Geometry check sheet. Reference: the model listing, model coordinates, mm. A direction names the side the tool comes from. Round coordinates to 2 decimals unless told otherwise and drop trailing zeros. Loops run counter-clockwise (first coordinate to the right, second up) from the corner with the lowest first, then second, coordinate; pieces in that order, holes last. Notation, with made-up numbers: (-5.75, 6) -> (23.25, 6) arc R15 ccw to (23.25, 14) -> close; hole circle Ø9 at (49, 24.5). An arc over 180 degrees is marked (long way). Use one line per item in the form item = value.
from build123d import *

# Parameters (mm, degrees)
F1_DEPTH = 63.5
F0_W     = 13.4667371243
F0_H     = 19.05
F2_DEPTH = 25.4
F3_DEPTH = 8.255
F5_R     = 5.08


with BuildPart() as f1:
    # F0 (on Front) → F1 (new body, symmetric)
    with BuildSketch(Plane.XZ):
        Polygon((-41.275, 9.525), (-41.275, -9.525), (41.275, -9.525), (41.275, 9.525), (22.225, 9.525), align=None)
    extrude(amount=F1_DEPTH, both=True)

    # F0 (on Front) → F2 (join, symmetric)
    with BuildSketch(Plane.XZ):
        with BuildLine():
            Line((22.225, 9.525), (41.275, 9.525))
            Line((41.275, 9.525), (41.275, 50.8))
            ThreePointArc((41.275, 50.8), (45.9246798487, 62.0253201513), (57.15, 66.675))
            Line((57.15, 66.675), (75.8414548727, 66.675))
            Line((75.8414548727, 66.675), (75.8414548727, 85.725))
            Line((75.8414548727, 85.725), (57.15, 85.725))
            ThreePointArc((57.15, 85.725), (32.4542956671, 75.4957043329), (22.225, 50.8))
            Line((22.225, 50.8), (22.225, 9.525))
        make_face()
        with Locations((82.5748234349, 76.2)):
            Rectangle(F0_W, F0_H)
    extrude(amount=F2_DEPTH, both=True)

    # F0 (on Front) → F3 (join, symmetric)
    with BuildSketch(Plane.XZ):
        with BuildLine():
            add(Edge.make_bspline(
                [(-41.275, 9.525), (-37.2192449868, 66.8318197131), (0, 89.7414088249), (75.8414548727, 85.725)],
                knots=[0, 0, 0, 0, 139.7236701563, 139.7236701563, 139.7236701563, 139.7236701563], degree=3))
            Line((-41.275, 9.525), (22.225, 9.525))
            Line((22.225, 9.525), (22.225, 50.8))
            ThreePointArc((22.225, 50.8), (32.4542956671, 75.4957043329), (57.15, 85.725))
            Line((57.15, 85.725), (75.8414548727, 85.725))
        make_face()
    extrude(amount=F3_DEPTH, both=True)

    # F0 (on Front) → F4 (revolve)
    with BuildSketch(Plane.XZ):
        Polygon((89.308191997, 97.7408438921), (89.308191997, 85.725), (89.308191997, 66.675), (89.308191997, 56.0535416007), (129.0989220142, 56.0535416007), (129.0989220142, 97.7408438921), align=None)
    revolve(axis=Axis((89.308191997, 0, 76.8971927464), (0, 0, 1)))

    # F5
    f5_edges = [f1.edges().sort_by_distance(p)[0] for p in [
        (41.275, 44.45, 9.525),
        (-41.275, 63.5, 0),
        (-41.275, -63.5, 0),
        (41.275, 63.5, 0),
        (41.275, -63.5, 0),
    ]]
    fillet(f5_edges, radius=F5_R)


solid = f1.part
1. Material ranges on line 1 along Z through (x, y) = (56, -20); line 2 along X through (y, z) = (15.5, -3) (3 decimals); line 3 along Z through (x, y) = (-27.5, -21) (3 decimals), recorded low to high.
Return value:
line_1 = 56.05 to 97.74
line_2 = -41.275 to 41.275
line_3 = -9.525 to 9.525
2. Section check C-C (x = 99). Record the boundary of the cut face in (y, z).
Return value:
outline = (-38.59, 56.05) -> (38.59, 56.05) -> (38.59, 97.74) -> (-38.59, 97.74) -> close
3. Section check D-D (y = 15). Record the boundary of the cut face in (x, z) (3 decimals), then the cut area to 3 significant figures.
Return value:
outline = (-41.275, -9.525) -> (41.275, -9.525) -> (41.275, 50.8) arc R15.875 cw to (52.453, 65.964) -> (52.453, 56.054) -> (126.163, 56.054) -> (126.163, 97.741) -> (52.453, 97.741) -> (52.453, 85.408) arc R34.925 ccw to (22.225, 50.8) -> (22.225, 9.525) -> (-41.275, 9.525) -> close
area = 6,100 mm2
4. Tool access check on faces 5 (the cylindrical face through (39.8, 62, 0.1)), 6 (the flat face through (41.275, -1, 14)), 7 (the flat face through (-5, 8.255, 40)), 8 (the flat face through (-5, -8.255, 40)). Record the directions out of +Z, -Z, +X, -X, +Y, -Y that give a thin tool (end or side, any length) a straight path to the whole face; none if there is none.
Return value:
face_5 = +Z, -Z, +X, +Y
face_6 = -Z, +X, +Y, -Y
face_7 = +Z, -X, +Y
face_8 = +Z, -X, -Y
5. Section check B-B (y = -21). Record the boundary of the cut face in (x, z) (3 decimals), then the cut area to 3 significant figures.
Return value:
outline = (-41.275, -9.525) -> (41.275, -9.525) -> (41.275, 50.8) arc R15.875 cw to (55.51, 66.59) -> (55.51, 56.054) -> (123.106, 56.054) -> (123.106, 97.741) -> (55.51, 97.741) -> (55.51, 85.686) arc R34.925 ccw to (22.225, 50.8) -> (22.225, 9.525) -> (-41.275, 9.525) -> close
area = 5,910 mm2
6. Gauge pin test, flat ends, axial feed: pin 1 (23 mm diameter, centred on x = 14.5, z = 41, fed in from -Y); pin 2 (5 mm diameter, centred on y = -13, z = 24, fed in from -X) (3 decimals); pin 3 (23 mm diameter, centred on x = 24, z = 56.5, fed in from +Y); pin 4 (12 mm diameter, centred on x = 55, y = -36, fed in from -Z). Record the tip position at first contact, or that the pin passes through.
Return value:
pin_1 = -25.4
pin_2 = 22.225
pin_3 = 25.4
pin_4 = through
7. Section check A-A (z = 2.5). Record the boundary of the cut face in (x, y) (3 decimals).
Return value:
outline = (-41.275, -58.42) arc R5.08 ccw to (-36.195, -63.5) -> (36.195, -63.5) arc R5.08 ccw to (41.275, -58.42) -> (41.275, 58.42) arc R5.08 ccw to (36.195, 63.5) -> (-36.195, 63.5) arc R5.08 ccw to (-41.275, 58.42) -> close
8. Mould release check, pull along X, two halves, no side actions. Record for faces 1 (the flat face through (90, 1, 56.054)), 2 (the cylindrical face through (44.047, -0.356, 59.762)), 3 (the cylindrical face through (32.73, -16.95, 75.77)), 4 (the cylindrical face through (39.747, 44.717, 8.076)): released by +X, released by -X, zero draft, split by the parting line, or undercut.
Return value:
face_1 = zero draft
face_2 = undercut
face_3 = released by -X
face_4 = released by +X
